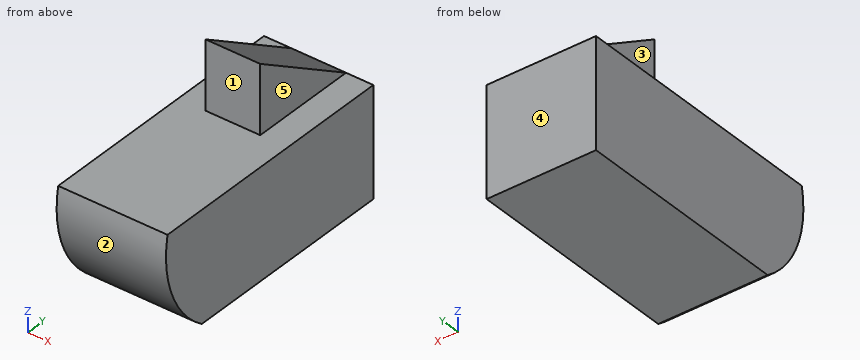
```python
from build123d import *

# Parameters (mm, degrees)
F1_DEPTH = 20
F3_DEPTH = 10


# Not quite as in the source:
# - a feature of the source that left no trace in its solid (it failed there, or was rolled back) is left out


with BuildPart() as f1:
    # F0 (on Right) → F1 (new body, symmetric)
    with BuildSketch(Plane.YZ):
        Polygon((-27.5, 18.3739837377), (-40, 18.3739837377), (-40, -21.6260162623), (40, -21.6260162623), (40, 18.3739837377), (11.153018102, 18.3739837377), (0, 18.3739837377), (-5, 18.3739837377), (-17.5, 18.3739837377), align=None)
        with BuildLine():
            Line((-40, -21.6260162623), (-40, 18.3739837377))
            Line((-40, 18.3739837377), (-50.9159490466, 18.3739837377))
            Line((-50.9159490466, 18.3739837377), (-55.972136481, 18.3739837377))
            ThreePointArc((-55.972136481, 18.3739837377), (-53.829536351, -3.9593330169), (-40, -21.6260162623))
        make_face()
    extrude(amount=F1_DEPTH, both=True)

    # F0 (on Right) → F3 (join, symmetric)
    with BuildSketch(Plane.YZ):
        Polygon((11.153018102, 18.3739837377), (40, 18.3739837377), (0, 43.3739837377), (0, 18.3739837377), align=None)
    extrude(amount=F3_DEPTH, both=True)


solid = f1.part
```
Could you check a few things on this model? Use its own coordinates, in mm. Face numbers are marked on the shaded views. A direction names the side the tool comes from. Round coordinates to 2 decimals unless told otherwise and drop trailing zeros. Loops run counter-clockwise (first coordinate to the right, second up) from the corner with the lowest first, then second, coordinate; pieces in that order, holes last. Notation, with made-up numbers: M -38,62.25 L 12,62.25 A19 ccw 12,66.25 Z; hole C 21.25,70 d11. An arc over 180 degrees is marked long. Answer as CSV lines item,"result".
1) Imagine slicing it at A-A on x = -4. List the corners of the cut face in (y, z) for me, and give its area (3 significant figures).
From the geometry:
outline,"M -55.97,18.37 A40 ccw -40,-21.63 L 40,-21.63 L 40,18.37 L 0,43.37 L 0,18.37 Z"
area,"4,200 mm^2"
2) For pin 1 Ø10 at (x, z) = (0.5, 32.5) entering from -Y; pin 2 Ø2 at (y, z) = (5, 19.5) entering from -X; pin 3 Ø3 at (x, y) = (14.5, 27.5) entering from +Z, each with a flat end and sliding along its axis, tell me the tip position at first contact or that it passes through.
From the geometry:
pin 1,"y = 0"
pin 2,"x = -10"
pin 3,"z = 18.37"
3) Imagine slicing it at C-C on z = -10. List the corners of the cut face in (x, y) for me.
From the geometry:
outline,"M -20,-50.8 L 20,-50.8 L 20,40 L -20,40 Z"
4) Which directions (+Z, -Z, +X, -X, +Y, -Y) give clear straight access to the entire face, cutting with the end or side of a thin tool? Please do the marked faces 1, 2, 3, 4 and 5.
From the geometry:
face 1,"+Z, +X, -X, -Y"
face 2,"+X, -X, -Y"
face 3,"+Z, -X, +Y, -Y"
face 4,"+Z, -Z, +X, -X, +Y"
face 5,"+Z, +X, +Y, -Y"
5) Imagine slicing it at D-D on x = 13. List the corners of the cut face in (y, z) for me, and give its area (3 significant figures).
From the geometry:
outline,"M -55.97,18.37 A40 ccw -40,-21.63 L 40,-21.63 L 40,18.37 Z"
area,"3,700 mm^2"
6) If I drill on probe 1 along Z at (x, y) = (-1.5, -25.5); probe 2 along X at (y, z) = (18.5, 30.5); probe 3 along Y at (x, z) = (11, 3.5), over which ranges is the centre line in solid material (lowest first)?
From the geometry:
probe 1,"-21.63 to 18.37"
probe 2,"-10 to 10"
probe 3,"-56 to 40"
7) Imagine slicing it at B-B on y = 27. List the corners of the cut face in (x, z) for me.
From the geometry:
outline,"M -20,-21.63 L 20,-21.63 L 20,18.37 L 10,18.37 L 10,26.5 L -10,26.5 L -10,18.37 L -20,18.37 Z"
